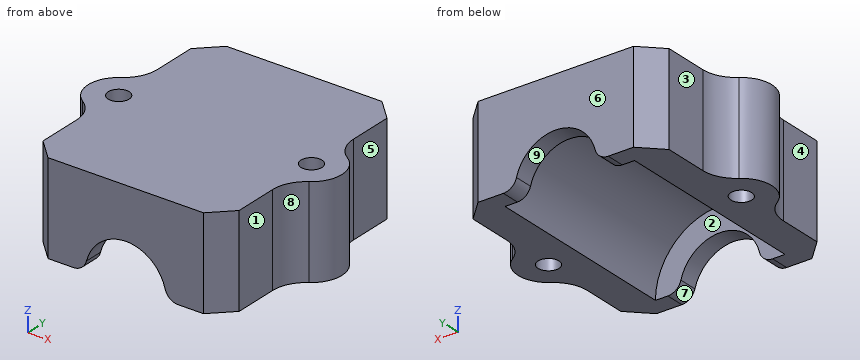
Autodesk Inventor part; units mm, degrees
ref_plane "YZ Plane" through (0, 0, 0) normal (1, 0, 0) x (0, 1, 0)
ref_plane "XZ Plane" through (0, 0, 0) normal (0, 1, 0) x (-1, 0, 0)
ref_plane "XY Plane" through (0, 0, 0) normal (0, 0, 1) x (1, 0, 0)
sketch "Szkic1" plane through (0, 0, 0) normal (0, 0, 1) x (1, 0, 0)
  line L0 (-13.3884, 18.62) -> (15.6116, 18.62)
  line L1 (15.6116, 18.62) -> (15.6116, -16.38)
  line L2 (15.6116, -16.38) -> (-13.3884, -16.38)
  line L3 (-13.3884, -16.38) -> (-13.3884, 18.62)
  arc A0 (-13.3884, 5.6124) -> (-13.3884, -3.3724) centre (-13.1267, 1.12) ccw
  arc A1 (15.6116, -3.3737) -> (15.6116, 5.6137) centre (15.3733, 1.12) ccw
  point P0 (0, 0)
  dimension "d2" = 35
  dimension "d5" = 28.5
  dimension "d6" = 29
  dimension "d7" = 17.5
  dimension "d8" = 17.5
  dimension "d9" = 9
  dimension "d10" = 9
extrude "Wyciągnięcie proste1" add sketch "Szkic1" along normal blind 13.5
hole "Otwór1" at (-13.1267, 1.12, 0) at (15.3733, 1.12, 0) direction (0, 0, 1) diameter 3.1 end through all
sketch "Szkic2" plane through (-13.3884, -16.38, 0) normal (0, -1, 0) x (1, 0, 0)
  line L0 (29, 0) -> (0, 0)
  line L1 (29, 0) -> (29, 13.5)
  line L2 (0, 13.5) -> (29, 13.5)
  line L3 (0, 0) -> (0, 13.5)
  circle A0 centre (14.5, 0) radius 9.575
  point P0 (13.3884, 0)
  dimension "d18" = 13.5
  dimension "d19" = 14.5
  dimension "d20" = 29
  dimension "d21" = 19.15
extrude "Wyciągnięcie proste2" cut sketch "Szkic2" against normal through all contours A0 L0 | L0 A0
sketch "Szkic3" plane through (-13.3884, -16.38, 13.5) normal (0, -1, 0) x (1, 0, 0)
  arc A0 (24.075, -13.5) -> (4.925, -13.5) centre (14.5, -13.5) ccw
  line L0 (29, -13.5) -> (24.075, -13.5)
  line L1 (29, -13.5) -> (29, 0)
  line L2 (0, 0) -> (29, 0)
  line L3 (0, -13.5) -> (0, 0)
  line L4 (4.925, -13.5) -> (0, -13.5)
  arc A1 (20.5, -13.5) -> (8.5, -13.5) centre (14.5, -13.5) ccw
  line L5 (0, -13.5) -> (4.925, -13.5)
  arc A2 (24.075, -13.5) -> (4.925, -13.5) centre (14.5, -13.5) ccw
  line L6 (4.925, -13.5) -> (24.075, -13.5)
  point P0 (13.3884, -13.5)
  dimension "d24" = 12
extrude "Wyciągnięcie proste3" add sketch "Szkic3" against normal blind 2.75 contours L6 A1 A0
sketch "Szkic4" plane through (-13.3884, 18.62, 13.5) normal (0, 1, 0) x (1, 0, 0)
  line L0 (8.5, 13.5) -> (4.925, 13.5)
  arc A0 (4.925, 13.5) -> (24.075, 13.5) centre (14.5, 13.5) ccw
  line L1 (24.075, 13.5) -> (20.5, 13.5)
  arc A1 (8.5, 13.5) -> (20.5, 13.5) centre (14.5, 13.5) ccw
  arc A2 (4.925, 13.5) -> (24.075, 13.5) centre (14.5, 13.5) ccw
  line L2 (0, 13.5) -> (4.925, 13.5)
  line L3 (0, 13.5) -> (0, 0)
  line L4 (29, 0) -> (0, 0)
  line L5 (29, 13.5) -> (29, 0)
  line L6 (24.075, 13.5) -> (29, 13.5)
  point P0 (13.3884, 13.5)
extrude "Wyciągnięcie proste4" add sketch "Szkic4" against normal blind 2.75 contours A1 L1 A0 L0
fillet "Zaokrąglenie1" radius 5 4 edges at (15.6116, 5.6137, 6.75) (15.6116, -3.3737, 6.75) (-13.3884, -3.3724, 6.75) (-13.3884, 5.6124, 6.75)
fillet "Zaokrąglenie2" radius 2 4 edges at (7.1116, -15.005, 0) (-4.8884, -15.005, 0) (7.1116, 17.245, 0) (-4.8884, 17.245, 0)
chamfer "Faza1" distance 3 angle 45 4 edges at (-13.3884, 18.62, 6.75) (15.6116, 18.62, 6.75) (-13.3884, -16.38, 6.75) (15.6116, -16.38, 6.75)
properties part number "3DP_ABS_Y_Axis_Linear_Bearing_Mount_Top"
Check sheet for the modelled part. Datum: model origin and axes. Units: mm. Face numbers are marked on the shaded views. A direction names the side the tool comes from. Round coordinates to 2 decimals unless told otherwise and drop trailing zeros. Order: outer loops, then holes, each group sorted by start corner. A loop starts at its lowest first (then second) coordinate and runs counter-clockwise, first axis right, second up. Notation, with made-up numbers: (46, -13.5) - (83, -13.5) arc R19 cw to (83, -0.5) - close; hole circle Ø6 at (71.5, 43.5). An arc over 180 degrees is marked (long way). Write item = value, one per line.
Q1. Section check C-C (z = 8.5). Record the boundary of the cut face in (x, y).
Computed:
outline = (-15.62, -2.63) arc R5 cw to (-13.39, -6.79) - (-13.39, -13.38) - (-10.39, -16.38) - (12.61, -16.38) - (15.61, -13.38) - (15.61, -6.81) arc R5 cw to (17.85, -2.63) arc R4.5 ccw to (17.85, 4.87) arc R5 cw to (15.61, 9.05) - (15.61, 15.62) - (12.61, 18.62) - (-10.39, 18.62) - (-13.39, 15.62) - (-13.39, 9.03) arc R5 cw to (-15.62, 4.87) arc R4.5 ccw to start; hole circle Ø3.1 at (-13.13, 1.12); hole (-3.3, -13.63) - (5.52, -13.63) - (5.52, 15.87) - (-3.3, 15.87) - close; hole circle Ø3.1 at (15.37, 1.12)
Q2. Section check A-A (y = 1.12). Record the boundary of the cut face in (x, z) (3 decimals), and give its area (3 significant figures).
Computed:
outline = (-17.627, 0) - (-14.677, 0) - (-14.677, 13.5) - (-17.627, 13.5) - close; (-11.577, 0) - (-8.463, 0) arc R9.575 cw to (10.687, 0) - (13.823, 0) - (13.823, 13.5) - (-11.577, 13.5) - close; (16.923, 0) - (19.873, 0) - (19.873, 13.5) - (16.923, 13.5) - close
area = 279 mm^2
Q3. Draft check along X on the marked faces 6, 7, 8 and 9. Enter one of: pulls with the +X half, pulls with the -X half, needs draft (parallel to the pull), parting line crosses it, or undercut.
Computed:
face_6 = needs draft
face_7 = undercut
face_8 = pulls with the +X half
face_9 = undercut
Q4. Section check B-B (z = 5.25). State how many separate pieces and enclosed holes the cut face has, and give its area (3 significant figures).
Computed:
separate_pieces = 2
enclosed_holes = 2
area = 543 mm^2
Q5. Tool access check on the marked faces 1, 2, 3, 4 and 5. Record the directions out of +Z, -Z, +X, -X, +Y, -Y that give a thin tool (end or side, any length) a straight path to the whole face; none if there is none.
Computed:
face_1 = +Z, -Z, +X, -Y
face_2 = -Z
face_3 = +Z, -Z, -X, +Y
face_4 = +Z, -Z, -X, -Y
face_5 = +Z, -Z, +X, +Y
Q6. Go/stop test with flat-tipped pins: pin 1 (1.5 mm diameter, centred on y = -3.5, z = 6.5, fed in from +X); pin 2 (5.5 mm diameter, centred on y = 13, z = 9, fed in from -X); pin 3 (2 mm diameter, centred on y = 9.5, z = 5, fed in from +X); pin 4 (4 mm diameter, centred on x = -13.13, y = 1.12, fed in from +Z). Record where each tip stops, or that it passes through.
Computed:
pin_1 = 17.69
pin_2 = -13.39
pin_3 = 15.64
pin_4 = 13.5
Q7. Section check D-D (x = -1). Record the boundary of the cut face in (y, z).
Computed:
outline = (-16.38, 5.62) - (-13.63, 5.62) - (-13.63, 9.34) - (15.87, 9.34) - (15.87, 5.62) - (18.62, 5.62) - (18.62, 13.5) - (-16.38, 13.5) - close
Q8. Thickness scan on line 1 along X through (y, z) = (-8, 11); line 2 along X through (y, z) = (3, 5); line 3 along Y through (x, z) = (14.5, 12.75). Record the ranges inside material, lowest first.
Computed:
line_1 = -13.39 to 15.61
line_2 = -17.22 to -7.05, 9.28 to 19.46
line_3 = -14.49 to -0.16, 2.4 to 16.73
